from build123d import *

# Parameters (mm, degrees)
ESQUISSE1_R             = 15
ESQUISSE1_R_2           = 4
BOSS_EXTRU_1_DEPTH      = 20
ENL_V_MAT_EXTRU_1_DEPTH = 8


with BuildPart() as part:
    # Esquisse1 → Boss.-Extru.1 (new body)
    with BuildSketch(Plane(origin=(0, 0, 0), x_dir=(0, 0, -1), z_dir=(1, 0, 0))):
        with Locations((-27.152557625, -173.602016712)):
            Circle(ESQUISSE1_R)
        with Locations((-27.152557625, -173.602016712)):
            Circle(ESQUISSE1_R_2, mode=Mode.SUBTRACT)
    extrude(amount=BOSS_EXTRU_1_DEPTH)

    # Esquisse2 → Enlèv. mat.-Extru.1 (cut)
    with BuildSketch(Plane.ZY):
        Polygon((21.82354936, -178.887374244), (29.065307384, -180.859752013), (34.394315649, -175.57439448), (32.48156589, -168.31665918), (25.239807867, -166.344281411), (19.910799602, -171.629638944), align=None)
    extrude(amount=-ENL_V_MAT_EXTRU_1_DEPTH, mode=Mode.SUBTRACT)


solid = part.part
Read the model definition and answer for the solid it produces. Units are mm, in the model's axes. A direction names the side the tool comes from. Round coordinates to 2 decimals unless told otherwise and drop trailing zeros. Write each loop counter-clockwise with the first axis right and the second up, starting at its lowest first coordinate (ties: lowest second). Pieces come first, ordered by that corner, then holes. Notation, with made-up numbers: (-11, 47.25) - (3, 47.25) arc R22 ccw to (3, 82.25) - close; hole circle Ø1 at (12.25, -19). An arc over 180 degrees is marked (long way). Use a Markdown table: item, result.
(1) Straight lines are drawn through the part: line 1 along Y through (x, z) = (6.75, 31.5) (3 decimals); line 2 along Y through (x, z) = (2, 22.75); line 3 along Z through (x, y) = (7.5, -171.25). For each, find the intervals that lie inside material, in ascending order. Write a range as [from, to].
Reported:
| item | result |
|---|---|
| line 1 | [-187.958, -178.445], [-168.049, -159.246] |
| line 2 | [-187.94, -179.14], [-168.81, -159.26] |
| line 3 | [12.34, 20.29], [33.25, 41.97] |
(2) The part is cut by section B-B (x = 1.5). Write down the section's boundary in (y, z).
Reported:
| item | result |
|---|---|
| outline | circle Ø30 at (-173.6, 27.15); hole (-180.86, 29.07) - (-178.89, 21.82) - (-171.63, 19.91) - (-166.34, 25.24) - (-168.32, 32.48) - (-175.57, 34.39) - close |
(3) The part is cut by section A-A (y = -174.25). Write down the section's boundary in (x, z), then the cut area to 3 significant figures.
Reported:
| item | result |
|---|---|
| outline | (0, 12.17) - (20, 12.17) - (20, 23.21) - (8, 23.21) - (8, 20.6) - (0, 20.6) - close; (0, 34.05) - (8, 34.05) - (8, 31.1) - (20, 31.1) - (20, 42.14) - (0, 42.14) - close |
| area | 397 mm2 |
(4) The part is cut by section C-C (z = 33.5). Write down the section's boundary in (x, y).
Reported:
| item | result |
|---|---|
| outline | (0, -187.19) - (20, -187.19) - (20, -160.01) - (0, -160.01) - (0, -172.18) - (8, -172.18) - (8, -176.46) - (0, -176.46) - close |
(5) Which of the six approach directions +Z, -Z, +X, -X, +Y, -Y give full straight-line access (tool end or side, diameter ignored) to faces 4 (the flat face through (0, -177, 21)), 5 (the flat face through (3.94, -168.95, 22.61))?
Reported:
| item | result |
|---|---|
| face 4 | +Z, -Z, -X, +Y, -Y |
| face 5 | -X |
(6) The part is cut by section D-D (y = -167.75). Write down the section's boundary in (x, z).
Reported:
| item | result |
|---|---|
| outline | (0, 13.34) - (20, 13.34) - (20, 40.96) - (0, 40.96) - (0, 30.4) - (8, 30.4) - (8, 23.82) - (0, 23.82) - close |
(7) The mould has two halves that part along Y. Classify faces 1 (the flat face through (3.944, -171.996, 33.451)), 2 (the cylindrical face through (9.86, -172.942, 42.138)), 3 (the flat face through (20, -177, 24)): released by +Y, released by -Y, zero draft, split by the parting line, or undercut.
Reported:
| item | result |
|---|---|
| face 1 | undercut |
| face 2 | split by the parting line |
| face 3 | zero draft |
(8) Each of these flat-tipped pins is pushed along its axis until it touches: pin 1 Ø10 at (x, z) = (14.5, 21.5) entering from -Y; pin 2 Ø8 at (x, y) = (8.5, -184.5) entering from -Z; pin 3 Ø10 at (x, y) = (10.5, -167) entering from +Z. Where does it stop, or does it pass through?
Reported:
| item | result |
|---|---|
| pin 1 | y = -188.59 |
| pin 2 | z = 13.83 |
| pin 3 | z = 42.07 |
